Verification items for the finished model (mm, model axes). Face numbers are marked on the shaded views. A direction names the side the tool comes from. Coordinates: 2 decimals unless noted, no trailing zeros. Write each loop counter-clockwise with the first axis right and the second up, starting at its lowest first coordinate (ties: lowest second). Pieces come first, ordered by that corner, then holes. Notation, with made-up numbers: (73, -17.5) -> (87, -17.5) arc R17 ccw to (87, -7.5) -> close; hole circle Ø7 at (-18, 54). An arc over 180 degrees is marked (long way). Answer in a Markdown table with one row per item.
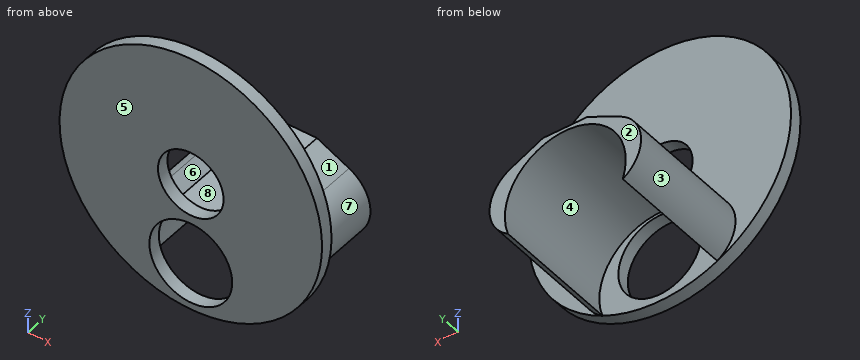
```python
from build123d import *

# Parameters (mm, degrees)
SKETCH1_R           = 20.6
BOSS_EXTRUDE1_DEPTH = 2
SKETCH2_R           = 5.15
CUT_EXTRUDE1_DEPTH  = 3
SKETCH3_R           = 6.5
CUT_EXTRUDE2_DEPTH  = 2
BOSS_EXTRUDE4_DEPTH = 20
FILLET2_R           = 6


with BuildPart() as part:
    # Sketch1 → Boss-Extrude1 (new body)
    with BuildSketch(Plane(origin=(0, 0, 0), x_dir=(1, 0, 0), z_dir=(0, 1, 0))):
        with Locations(Location((0, 0, 0), (0, 0, 270))):
            Circle(SKETCH1_R)
    extrude(amount=BOSS_EXTRUDE1_DEPTH)

    # Sketch2 → Cut-Extrude1 (cut)
    with BuildSketch(Plane(origin=(0, 2, 0), x_dir=(1, 0, 0), z_dir=(0, 1, 0))):
        with Locations(Location((0, 0, 0), (0, 0, 270))):
            Circle(SKETCH2_R)
    extrude(amount=-CUT_EXTRUDE1_DEPTH, mode=Mode.SUBTRACT)

    # Sketch3 → Cut-Extrude2 (cut)
    with BuildSketch(Plane(origin=(0, 2, 0), x_dir=(1, 0, 0), z_dir=(0, 1, 0))):
        with Locations(Location((0, 13, 0), (0, 0, 270))):
            Circle(SKETCH3_R)
    extrude(amount=-CUT_EXTRUDE2_DEPTH, mode=Mode.SUBTRACT)

    # Sketch4 → Boss-Extrude4 (add)
    with BuildSketch(Plane(origin=(0, 2, 0), x_dir=(1, 0, 0), z_dir=(0, 1, 0))):
        with BuildLine():
            Line((-16.743954133, 12), (-3.5, 5.5))
            Line((-3.5, 5.5), (3.5, 5.5))
            Line((3.5, 5.5), (16.743954133, 12))
            ThreePointArc((16.743954133, 12), (13.279606143, 15.748398671), (9, 18.529975715))
            ThreePointArc((9, 18.529975715), (0, 6.042759079), (-9, 18.529975715))
            ThreePointArc((-9, 18.529975715), (-13.279606143, 15.748398671), (-16.743954133, 12))
        make_face()
    extrude(amount=BOSS_EXTRUDE4_DEPTH)

    # Fillet2
    # the kernel refuses this fillet: 6 mm, written as the material it takes off along each edge
    with BuildSketch(Plane(origin=(16.743954133, 2, -12), x_dir=(-0.7761796310564387, 0, -0.6305118399626535), z_dir=(0, 1, 0))) as fillet2_piece_1:
        with BuildLine():
            CenterArc((9.278744028, 5.78779133), FILLET2_R, 155.229237023, 130.054584679)
            Line((3.830795632, 8.301724161), (0, 0))
            ThreePointArc((0, 0), (5.430174062, -0.728583099), (10.860348123, 0))
        make_face()
    extrude(amount=47.150870308, mode=Mode.SUBTRACT)
    with BuildSketch(Plane(origin=(-16.743954133, 2, -12), x_dir=(0.7761796310564387, 0, -0.6305118399626534), z_dir=(0, 1, 0))) as fillet2_piece_2:
        with BuildLine():
            CenterArc((9.278744028, -5.78779133), FILLET2_R, 74.716178298, 130.054584679)
            Line((3.830795632, -8.301724161), (0, 0))
            ThreePointArc((0, 0), (5.430174062, 0.728583099), (10.860348123, 0))
        make_face()
    extrude(amount=47.150870308, mode=Mode.SUBTRACT)


solid = part.part
```
1. Thickness scan on line 1 (Y direction, x = 10, z = 1); line 2 (X direction, y = 1.5, z = -13); line 3 (Z direction, x = 0, y = 9.75). Record the ranges inside material, lowest first. Write a range as from..to.
Geometry says:
| item | result |
|---|---|
| line 1 | 0..2 |
| line 2 | -15.98..-6.5, 6.5..15.98 |
| line 3 | -6.04..-5.5 |
2. Mould release check, pull along X, two halves, no side actions. Record for the marked faces 1, 2, 3 and 4: released by +X, released by -X, zero draft, split by the parting line, or undercut.
Geometry says:
| item | result |
|---|---|
| face 1 | released by +X |
| face 2 | zero draft |
| face 3 | released by -X |
| face 4 | undercut |
3. Section check A-A, the plane z = 0. Record the boundary of the cut face in (x, y).
Geometry says:
| item | result |
|---|---|
| outline | (-20.6, 0) -> (-5.15, 0) -> (-5.15, 2) -> (-20.6, 2) -> close; (5.15, 0) -> (20.6, 0) -> (20.6, 2) -> (5.15, 2) -> close |
4. Depth check by flat-ended pin: P1, Ø2, axis at x = -5, y = 6.5, coming from the +Z side; P2, Ø10, axis at x = -2, z = 14, coming from the +Y side; P3, Ø3.5, axis at x = 1, y = 9, coming from the +Z side. Enter the tip coordinate at first touch or a pass-through.
Geometry says:
| item | result |
|---|---|
| P1 | z = -5.75 |
| P2 | y = 2 |
| P3 | z = -5.5 |
5. Section check C-C, the plane y = 16.5. Record the boundary of the cut face in (x, z).
Geometry says:
| item | result |
|---|---|
| outline | (-9.02, -18.48) arc R9.49 cw (long way) to (9.02, -18.48) arc R6 ccw to (8.54, -7.97) -> (3.5, -5.5) -> (-3.5, -5.5) -> (-8.54, -7.97) arc R6 ccw to start |
6. Section check D-D, the plane z = -11.5. Record the boundary of the cut face in (x, y).
Geometry says:
| item | result |
|---|---|
| outline | (-17.09, 0) -> (-6.32, 0) -> (-6.32, 2) -> (-8.59, 2) -> (-8.59, 22) -> (-11.6, 22) -> (-11.6, 2) -> (-17.09, 2) -> close; (6.32, 0) -> (17.09, 0) -> (17.09, 2) -> (11.6, 2) -> (11.6, 22) -> (8.59, 22) -> (8.59, 2) -> (6.32, 2) -> close |
7. Tool access check on the marked faces 5, 6, 7 and 8. Record the directions out of +Z, -Z, +X, -X, +Y, -Y that give a thin tool (end or side, any length) a straight path to the whole face; none if there is none.
Geometry says:
| item | result |
|---|---|
| face 5 | +Z, -Z, +X, -X, -Y |
| face 6 | +Z, -X, +Y |
| face 7 | +X, +Y |
| face 8 | +Z, +X, -X, +Y |
8. Section check B-B, the plane x = -4. Record the boundary of the cut face in (y, z).
Geometry says:
| item | result |
|---|---|
| outline | (0, -20.21) -> (2, -20.21) -> (2, -18.12) -> (0, -18.12) -> close; (0, -7.88) -> (2, -7.88) -> (2, -6.93) -> (22, -6.93) -> (22, -5.75) -> (2, -5.75) -> (2, -3.24) -> (0, -3.24) -> close; (0, 3.24) -> (2, 3.24) -> (2, 20.21) -> (0, 20.21) -> close |
